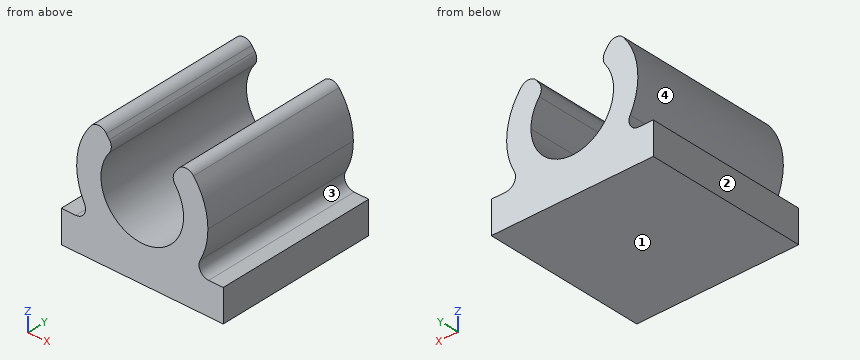
```python
from build123d import *

# Parameters (mm, degrees)
F1_DEPTH = 10
F2_R     = 0.6
F3_R     = 0.6


with BuildPart() as f1:
    # F0 (on Front) → F1 (new body)
    with BuildSketch(Plane.XZ):
        with BuildLine():
            Line((2.934854861, 2), (-2.934854861, 2))
            ThreePointArc((-2.934854861, 2), (0, 0.7409007408), (2.934854861, 2))
        make_face()
        with BuildLine():
            Line((-2.934854861, 2), (-5, 2))
            Line((-5, 2), (-5, 0))
            Line((-5, 0), (5, 0))
            Line((5, 0), (5, 2))
            Line((5, 2), (2.934854861, 2))
            ThreePointArc((2.934854861, 2), (0, 0.7409007408), (-2.934854861, 2))
        make_face()
        with BuildLine():
            ThreePointArc((-2.6329280886, 7.8682680702), (-4.0446500812, 4.9990010065), (-2.934854861, 2))
            Line((-2.934854861, 2), (2.934854861, 2))
            ThreePointArc((2.934854861, 2), (3.7608949857, 3.288180239), (4.05, 4.7909007408))
            ThreePointArc((4.05, 4.7909007408), (3.6787130058, 6.4848814433), (2.6329280886, 7.8682680702))
            Line((2.6329280886, 7.8682680702), (1.7395072673, 6.6554689125))
            ThreePointArc((1.7395072673, 6.6554689125), (2.3386153523, 5.8074528714), (2.55, 4.7909007408))
            ThreePointArc((2.55, 4.7909007408), (-1.0165521306, 2.4522853885), (-1.7395072673, 6.6554689125))
            Line((-1.7395072673, 6.6554689125), (-2.6329280886, 7.8682680702))
        make_face()
    extrude(amount=F1_DEPTH)

    # F2
    f2_edges = [f1.edges().sort_by_distance(p)[0] for p in [
        (1.739507, -5, 6.655469),
        (-1.739507, -5, 6.655469),
        (-2.632928, -5, 7.868268),
        (2.632928, -5, 7.868268),
    ]]
    fillet(f2_edges, radius=F2_R)

    # F3
    f3_edges = [f1.edges().sort_by_distance(p)[0] for p in [
        (2.934855, -5, 2),
        (-2.934855, -5, 2),
    ]]
    fillet(f3_edges, radius=F3_R)


solid = f1.part
```
Check sheet for the modelled part. Datum: model origin and axes. Units: mm. Face numbers are marked on the shaded views. Round coordinates to 2 decimals unless told otherwise and drop trailing zeros. Loops run counter-clockwise (first coordinate to the right, second up) from the corner with the lowest first, then second, coordinate; pieces in that order, holes last. Notation, with made-up numbers: (-20, 16.5) - (1, 16.5) arc R21 ccw to (1, 38.5) - close; hole circle Ø9 at (80.25, 88). An arc over 180 degrees is marked (long way). Answer as a JSON object with one key per item and string values. Group by question number.
Q1. Mould release check, pull along Z, two halves, no side actions. Record for the marked faces 1, 2, 3 and 4: released by +Z, released by -Z, zero draft, split by the parting line, or undercut.
Q2. Sectioned sample at D-D, the plane y = -8.75. Enter the section's corners in (x, z).
Q3. Sectioned sample at C-C, the plane x = 0. Enter the section's corners in (y, z), plus the area to 3 significant figures.
Q4. Scan lines: line 1 along Z through (x, y) = (0, -6); line 2 along X through (y, z) = (-8.25, 3); line 3 along X through (y, z) = (-2, 5). Record each from-to range of solid material in increasing order. Write a range as [from, to].
Q5. Sectioned sample at B-B, the plane z = 3.5. Enter the section's corners in (x, y).
Q6. Sectioned sample at A-A, the plane x = -3.75. Enter the section's corners in (y, z).
Q7. Gauge pin test, flat end, axial feed: P1, Ø0.7, axis at x = -4.5, y = -6.5, coming from the +Z side. Record the tip position at first contact, or that the pin passes through.
Solution:
{
 "1": {"face 1": "released by -Z", "face 2": "zero draft", "face 3": "undercut", "face 4": "undercut"},
 "2": {"outline": "(-5, 0) - (5, 0) - (5, 2) - (4.1, 2) arc R0.6 cw to (3.57, 2.88) arc R4.05 ccw to (3.17, 7.32) arc R0.6 ccw to (2.21, 7.3) - (2.03, 7.05) arc R0.6 ccw to (2.03, 6.33) arc R2.55 cw (long way) to (-2.03, 6.33) arc R0.6 ccw to (-2.03, 7.05) - (-2.21, 7.3) arc R0.6 ccw to (-3.17, 7.32) arc R4.05 ccw to (-3.57, 2.88) arc R0.6 cw to (-4.1, 2) - (-5, 2) - close"},
 "3": {"outline": "(-10, 0) - (0, 0) - (0, 2.24) - (-10, 2.24) - close", "area": "22.4 mm²"},
 "4": {"line 1": "z = [0, 2.24]", "line 2": "x = [-3.63, -1.82], [1.82, 3.63]", "line 3": "x = [-4.04, -2.54], [2.54, 4.04]"},
 "5": {"outline": "(-3.84, -10) - (-2.2, -10) - (-2.2, 0) - (-3.84, 0) - close; (2.2, -10) - (3.84, -10) - (3.84, 0) - (2.2, 0) - close"},
 "6": {"outline": "(-10, 0) - (0, 0) - (0, 2.11) - (-10, 2.11) - close; (-10, 3.26) - (0, 3.26) - (0, 6.32) - (-10, 6.32) - close"},
 "7": {"P1": "stops at z = 2"}
}
